Design review of the part built by this model. Coordinates are the model's own, in mm. Face numbers are marked on the shaded views. A direction names the side the tool comes from. Coordinates: 2 decimals unless noted, no trailing zeros. Loops run counter-clockwise (first coordinate to the right, second up) from the corner with the lowest first, then second, coordinate; pieces in that order, holes last. Notation, with made-up numbers: (39, 87) - (45, 87) arc R14 cw to (45, 109) - close; hole circle Ø9 at (57, 27.5). An arc over 180 degrees is marked (long way). One line per question, with ' | ' between items.
from build123d import *

# Parameters (mm, degrees)
BOSS_EXTRUDE1_DEPTH = 2.05
BOSS_EXTRUDE2_START = 2.05
BOSS_EXTRUDE2_DEPTH = 4.1
FILLET1_R           = 10
SKETCH2_R           = 1.66
CUT_EXTRUDE1_DEPTH  = 30.406512034
SKETCH2_3_R         = 4.275
SKETCH2_3_R_2       = 1.66
CUT_EXTRUDE2_DEPTH  = 1.05
SKETCH3_R           = 1.325
CUT_EXTRUDE3_DEPTH  = 30.406512034
CUT_EXTRUDE4_DEPTH  = 30.406512034
CUT_EXTRUDE5_DEPTH  = 4.42
SKETCH6_R           = 3
CUT_EXTRUDE6_DEPTH  = 3.57
SKETCH7_R           = 1.76
BOSS_EXTRUDE3_DEPTH = 2


with BuildPart() as part:
    # Sketch1 → Boss-Extrude1 (new body)
    with BuildSketch(Plane(origin=(0, 0, 0), x_dir=(1, 0, 0), z_dir=(0, 1, 0))):
        with BuildLine():
            ThreePointArc((7.485, 0), (6.484364849, 3.738748119), (3.75, 6.477864231))
            Line((3.75, 6.477864231), (3.75, 0))
            ThreePointArc((3.75, 0), (0, -3.75), (-3.75, 0))
            Line((-3.75, 0), (-3.75, 6.477864231))
            ThreePointArc((-3.75, 6.477864231), (-3.738748119, -6.484364849), (7.485, 0))
        make_face()
        with BuildLine():
            Line((3.75, 0), (3.75, 6.477864231))
            ThreePointArc((3.75, 6.477864231), (0, 7.485), (-3.75, 6.477864231))
            Line((-3.75, 6.477864231), (-3.75, 0))
            ThreePointArc((-3.75, 0), (0, -3.75), (3.75, 0))
        make_face()
        with BuildLine():
            Line((-3, 24.015), (-3, 19.955))
            ThreePointArc((-3, 19.955), (0, 16.955), (3, 19.955))
            Line((3, 19.955), (3, 24.015))
            ThreePointArc((3, 24.015), (0, 27.015), (-3, 24.015))
        make_face()
    extrude(amount=BOSS_EXTRUDE1_DEPTH)

    # Sketch1<3> → Boss-Extrude2 (add)
    # profile 1 of 6: a face of its own
    with BuildSketch(Plane(origin=(0, 0, 0), x_dir=(1, 0, 0), z_dir=(0, 1, 0)).offset(BOSS_EXTRUDE2_START)):
        with BuildLine():
            ThreePointArc((7.485, 0), (6.484364849, 3.738748119), (3.75, 6.477864231))
            Line((3.75, 6.477864231), (3.75, 0))
            ThreePointArc((3.75, 0), (0, -3.75), (-3.75, 0))
            Line((-3.75, 0), (-3.75, 6.477864231))
            ThreePointArc((-3.75, 6.477864231), (-3.738748119, -6.484364849), (7.485, 0))
        make_face()
    # profile 2 of 6: a face of its own
    with BuildSketch(Plane(origin=(0, 0, 0), x_dir=(1, 0, 0), z_dir=(0, 1, 0)).offset(BOSS_EXTRUDE2_START)):
        with BuildLine():
            Line((3.75, 0), (3.75, 6.477864231))
            ThreePointArc((3.75, 6.477864231), (0, 7.485), (-3.75, 6.477864231))
            Line((-3.75, 6.477864231), (-3.75, 0))
            ThreePointArc((-3.75, 0), (0, -3.75), (3.75, 0))
        make_face()
    # profile 3 of 6: a face of its own
    with BuildSketch(Plane(origin=(0, 0, 0), x_dir=(1, 0, 0), z_dir=(0, 1, 0)).offset(BOSS_EXTRUDE2_START)):
        with BuildLine():
            ThreePointArc((7.485, 0), (6.484364849, 3.738748119), (3.75, 6.477864231))
            Line((3.75, 6.477864231), (3.75, 0))
            ThreePointArc((3.75, 0), (0, -3.75), (-3.75, 0))
            Line((-3.75, 0), (-3.75, 6.477864231))
            ThreePointArc((-3.75, 6.477864231), (-3.738748119, -6.484364849), (7.485, 0))
        make_face()
    # profile 4 of 6: a face of its own
    with BuildSketch(Plane(origin=(0, 0, 0), x_dir=(1, 0, 0), z_dir=(0, 1, 0)).offset(BOSS_EXTRUDE2_START)):
        with BuildLine():
            Line((3.75, 0), (3.75, 6.477864231))
            ThreePointArc((3.75, 6.477864231), (0, 7.485), (-3.75, 6.477864231))
            Line((-3.75, 6.477864231), (-3.75, 0))
            ThreePointArc((-3.75, 0), (0, -3.75), (3.75, 0))
        make_face()
    # profile 5 of 6: a face of its own
    with BuildSketch(Plane(origin=(0, 0, 0), x_dir=(1, 0, 0), z_dir=(0, 1, 0)).offset(BOSS_EXTRUDE2_START)):
        with BuildLine():
            Line((3.75, 6.477864231), (3.75, 24.015))
            ThreePointArc((3.75, 24.015), (0, 27.765), (-3.75, 24.015))
            Line((-3.75, 24.015), (-3.75, 6.477864231))
            ThreePointArc((-3.75, 6.477864231), (0, 7.485), (3.75, 6.477864231))
        make_face()
        with BuildLine():
            ThreePointArc((-3, 24.015), (0, 27.015), (3, 24.015))
            Line((3, 24.015), (3, 19.955))
            ThreePointArc((3, 19.955), (0, 16.955), (-3, 19.955))
            Line((-3, 19.955), (-3, 24.015))
        make_face(mode=Mode.SUBTRACT)
    # profile 6 of 6: a face of its own
    with BuildSketch(Plane(origin=(0, 0, 0), x_dir=(1, 0, 0), z_dir=(0, 1, 0)).offset(BOSS_EXTRUDE2_START)):
        with BuildLine():
            Line((-3, 24.015), (-3, 19.955))
            ThreePointArc((-3, 19.955), (0, 16.955), (3, 19.955))
            Line((3, 19.955), (3, 24.015))
            ThreePointArc((3, 24.015), (0, 27.015), (-3, 24.015))
        make_face()
    extrude(amount=BOSS_EXTRUDE2_DEPTH)

    # Fillet1
    fillet1_edges = [part.edges().sort_by_distance(p)[0] for p in [
        (-3.75, 4.1, -6.477864231),
        (3.75, 4.1, -6.477864231),
    ]]
    fillet(fillet1_edges, radius=FILLET1_R)

    # Sketch2 → Cut-Extrude1 (cut, through all)
    with BuildSketch(Plane(origin=(0, 6.15, 0), x_dir=(1, 0, 0), z_dir=(0, 1, 0))):
        with Locations(Location((0, 0, 0), (0, 0, 270))):
            Circle(SKETCH2_R)
    extrude(amount=-CUT_EXTRUDE1_DEPTH, mode=Mode.SUBTRACT)

    # Sketch2<3> → Cut-Extrude2 (cut)
    with BuildSketch(Plane(origin=(0, 6.15, 0), x_dir=(1, 0, 0), z_dir=(0, 1, 0))):
        with Locations(Location((0, 0, 0), (0, 0, 270))):
            Circle(SKETCH2_3_R)
        with Locations(Location((0, 0, 0), (0, 0, 270))):
            Circle(SKETCH2_3_R_2, mode=Mode.SUBTRACT)
    extrude(amount=-CUT_EXTRUDE2_DEPTH, mode=Mode.SUBTRACT)

    # Sketch3 → Cut-Extrude3 (cut, through all)
    with BuildSketch(Plane(origin=(0, 0, 0), x_dir=(-1, 0, 0), z_dir=(0, -1, 0))):
        with Locations(Location((0, 19.94, 0), (0, 0, 90))):
            Circle(SKETCH3_R)
        with Locations(Location((0, 24.09, 0), (0, 0, 90))):
            Circle(SKETCH3_R)
    extrude(amount=-CUT_EXTRUDE3_DEPTH, mode=Mode.SUBTRACT)

    # Sketch4 → Cut-Extrude4 (cut, symmetric)
    with BuildSketch(Plane.XY):
        Polygon((-23.349611589, -29.172910653), (5.823299064, 0), (7.485, 1.661700936), (36.657910653, 30.834611589), (95.003731959, -27.511209717), (34.996209717, -87.518731959), align=None)
    cut_extrude4 = extrude(amount=CUT_EXTRUDE4_DEPTH, both=True, mode=Mode.SUBTRACT)

    # Mirror1: Cut-Extrude4 across plane
    add(cut_extrude4.mirror(Plane(origin=(0, 0, 0), x_dir=(0, 0, 1), z_dir=(1, 0, 0))), mode=Mode.SUBTRACT)

    # Sketch5 → Cut-Extrude5 (cut)
    with BuildSketch(Plane.XZ):
        with BuildLine():
            Line((21.72046725, -1.797403589), (4.635, -1.797403589))
            ThreePointArc((4.635, -1.797403589), (3.574339828, -2.236743417), (3.135, -3.297403589))
            Line((3.135, -3.297403589), (3.135, -6.297403589))
            ThreePointArc((3.135, -6.297403589), (3.574339828, -7.35806376), (4.635, -7.797403589))
            Line((4.635, -7.797403589), (21.72046725, -7.797403589))
            Line((21.72046725, -7.797403589), (21.72046725, -1.797403589))
        make_face()
        with BuildLine():
            Line((-4.635, 1.797403589), (-13.906337827, 1.797403589))
            Line((-13.906337827, 1.797403589), (-13.906337827, 10.507844077))
            Line((-13.906337827, 10.507844077), (-3.135, 10.507844077))
            Line((-3.135, 10.507844077), (-3.135, 3.297403589))
            ThreePointArc((-3.135, 3.297403589), (-3.574339828, 2.236743417), (-4.635, 1.797403589))
        make_face()
    extrude(amount=-CUT_EXTRUDE5_DEPTH, mode=Mode.SUBTRACT)

    # Sketch6 → Cut-Extrude6 (cut)
    with BuildSketch(Plane.XZ):
        with Locations(Location((0, 0, 0), (0, 0, 270))):
            Circle(SKETCH6_R)
    extrude(amount=-CUT_EXTRUDE6_DEPTH, mode=Mode.SUBTRACT)

    # Sketch7 → Boss-Extrude3 (add)
    with BuildSketch(Plane.ZY.offset(3.135)):
        with Locations(Location((4.997403589, 1.92, 0), (0, 0, 164.996295671))):
            Circle(SKETCH7_R)
    extrude(amount=BOSS_EXTRUDE3_DEPTH)


solid = part.part
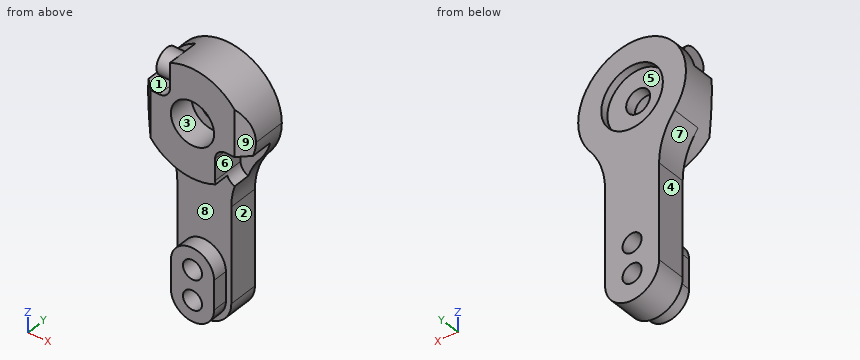
Q1. Take a section at A-A (y = 0.5). Give the boundary of the cut face in (x, z) (3 decimals), plus the area to 3 significant figures.
Returned:
outline: (-6.323, -4.005) arc R7.485 ccw to (3.209, -6.762) arc R1.5 cw to (3.135, -6.297) - (3.135, -3.297) arc R1.5 cw to (4.635, -1.797) - (6.323, -1.797) - (6.323, 4.005) arc R7.485 ccw to (-3.135, 6.797) - (-3.135, 6.037) - (-5.135, 6.037) - (-5.135, 3.958) - (-3.135, 3.958) - (-3.135, 3.297) arc R1.5 cw to (-4.635, 1.797) - (-6.323, 1.797) - close; (-3, -24.015) arc R3 ccw to (3, -24.015) - (3, -19.955) arc R3 ccw to (-3, -19.955) - close; hole circle Ø6 at (0, 0); hole circle Ø2.65 at (0, -24.09); hole circle Ø2.65 at (0, -19.94) | area: 157 mm²
Q2. Take a section at D-D (z = -16.5). Give the boundary of the cut face in (x, y), plus the area to 4 significant figures.
Returned:
outline: (-3.75, 2.05) - (3.75, 2.05) - (3.75, 6.15) - (-3.75, 6.15) - close | area: 30.75 mm²
Q3. Take a section at C-C (y = 5.5). Give the boundary of the cut face in (x, z) (3 decimals), plus the area to 3 significant figures.
Returned:
outline: (-5.886, -4.624) arc R10 cw to (-3.75, -10.801) - (-3.75, -24.015) arc R3.75 ccw to (3.75, -24.015) - (3.75, -10.801) arc R10 cw to (5.886, -4.624) arc R7.485 ccw (long way) to start; hole circle Ø8.55 at (0, 0); hole circle Ø2.65 at (0, -24.09); hole circle Ø2.65 at (0, -19.94) | area: 260 mm²
Q4. To check wall thickness, follow line 1 along X through (y, z) = (1.5, -24.09) (3 decimals); line 2 along Z through (x, y) = (-1, 4.25) (3 decimals); line 3 along Z through (x, y) = (-2.5, 1.75). State the ranges of each line that lie inside material, in increasing order.
Returned:
line 1: x = -2.999 to -1.325, 1.325 to 2.999 | line 2: z = -27.629 to -24.959, -23.221 to -20.809, -19.071 to -1.325, 1.325 to 7.418 | line 3: z = -25.67 to -18.3, -7.06 to -1.66, 1.66 to 7.06
Q5. Tool access review of the marked faces 1, 2, 3, 4 and 5: name each direction out of +Z, -Z, +X, -X, +Y, -Y from which nothing blocks a thin tool from reaching the whole face with its end or side.
Returned:
face 1: -X, -Y | face 2: -Z, +X, +Y, -Y | face 3: -Y | face 4: -Z, -X, +Y, -Y | face 5: +Y
Q6. Take a section at B-B (x = 0). State how many separate pieces and enclosed holes the cut face has, plus the area to 3 significant figures.
Returned:
separate pieces: 4 | enclosed holes: 0 | area: 128 mm²
Q7. Draft analysis for pull direction Z (two halves, no side actions). For the marked faces 6, 7, 8 and 9, state which applies: +Z half, -Z half, draft (parallel to the pull), parting line (faces both ways), or undercut.
Returned:
face 6: undercut | face 7: -Z half | face 8: undercut | face 9: draft
Q8. For pin 1 (1.3 mm diameter, centred on x = -6, y = 1.5, fed in from +Z); pin 2 (3 mm diameter, centred on y = 5, z = -13, fed in from +X); pin 3 (3 mm diameter, centred on y = 1.5, z = 5, fed in from -X) (3 decimals), all flat-tipped, find the tip position at first contact; note any pin that passes through.
Returned:
pin 1: stops at z = 1.8 | pin 2: stops at x = 3.75 | pin 3: stops at x = -5.135
